Geometry: final body of the model. Coordinates: model frame, mm. Face numbers are marked on the shaded views. A direction names the side the tool comes from. Give positions to 0.01 mm unless a question says otherwise; leave off trailing zeros. Write each loop counter-clockwise with the first axis right and the second up, starting at its lowest first coordinate (ties: lowest second). Pieces come first, ordered by that corner, then holes. Notation, with made-up numbers: M 62.25,-10.75 L 93.25,-10.75 A28 ccw 93.25,14.25 Z; hole C -15,17.5 d7. An arc over 180 degrees is marked long. Use one line per item in the form item = value. Start each with the question number.
Item 1: Section query D-D on x = 15.75. Return loops of the section in (y, z).
Item 2: Access query for the marked faces 5, 6, 7, 8 and 9. Directions: +Z, -Z, +X, -X, +Y, -Y. A direction counts if a zero-diameter tool reaches every point of the face in a straight line with its end or side. Return the directions, or none.
Item 3: Section query C-C on x = 2.75. Return loops of the section in (y, z).
Item 4: Pull-direction query (X, two-part tool) for the marked faces 1, 2, 3 and 4; classes: released by +X, released by -X, zero draft, split by the parting line, or undercut.
Item 5: Contact query for flat-ended pins moving along their axis: P1, Ø1.5, axis at x = 16, z = 10.5, coming from the -Y side; P2, Ø7, axis at y = 10.5, z = 9, coming from the -X side; P3, Ø10.5, axis at y = 11, z = 10.5, coming from the +X side. Output: stop coordinate, or through.
Item 6: Material intervals for line 1 along X through (y, z) = (22.5, 4); line 2 along Y through (x, z) = (9.25, 3.25); line 3 along X through (y, z) = (7, 2) (3 decimals), sorted ascending. Write a range as from..to.
Item 7: Section query A-A on y = 23.5. Return loops of the section in (x, z), then the cut area to 3 significant figures.
from build123d import *

# Parameters (mm, degrees)
F0_W        = 7.366
F0_H        = 10.16
F1_DEPTH    = 19.05
F2_T4_DEPTH = 19.05
F2_T9_DEPTH = 19.05
F3_SIZE     = 2.54
F4_SIZE     = 6.35
F5_R        = 1.016


# Not quite as in the source:
# - a fillet or chamfer that OpenCascade refuses, or shapes differently, is made with other operations: its cross-section is extruded or revolved along the edge and cut away or added


with BuildPart() as f1:
    # F0 (on Top) → F1 (new body)
    with BuildSketch(Plane.XY):
        Polygon((0, 20.4722661398), (0, 0), (3.175, 0), (3.175, 10.16), (3.175, 11.43), (8.255, 11.43), (13.335, 11.43), (13.335, 0), (16.51, 0), (16.51, 20.4722661398), (19.3675, 20.4722661398), (19.3675, 33.02), (16.1925, 33.02), (16.1925, 20.32), (8.255, 20.32), (0.3175, 20.32), (0.3175, 33.02), (-2.8575, 33.02), (-2.8575, 20.4722661398), align=None)
        with Locations((6.858, 5.08)):
            Rectangle(F0_W, F0_H)
    extrude(amount=F1_DEPTH)

    # F2: chamfer of 5.08 on 2 edges, made by hand


with BuildPart() as f2_tool2:
    # F2_s3 → F2_t4 (new body)
    with BuildSketch(Plane.XY):
        Polygon((-5.08, 20.4722661398), (0, 15.3922661398), (0, 20.4722661398), align=None)
    extrude(amount=F2_T4_DEPTH)

    split(bisect_by=Plane.YZ.offset(-2.8575), keep=Keep.TOP)


with BuildPart() as f1_1:
    add(f1.part)

    # F2_t1: union F2_tool2
    add(f2_tool2.part)


with BuildPart() as f2_tool7:
    # F2_s8 → F2_t9 (new body)
    with BuildSketch(Plane.XY):
        Polygon((16.51, 15.3922661398), (21.59, 20.4722661398), (16.51, 20.4722661398), align=None)
    extrude(amount=F2_T9_DEPTH)

    split(bisect_by=Plane.YZ.offset(19.3675), keep=Keep.BOTTOM)


with BuildPart() as f1_2:
    add(f1_1.part)

    # F2_t6: union F2_tool7
    add(f2_tool7.part)

    # F3
    f3_edges = [f1_2.edges().sort_by_distance(p)[0] for p in [
        (16.51, 0, 9.525),
        (19.3675, 33.02, 9.525),
    ]]
    chamfer(f3_edges, length=F3_SIZE)

    # F4
    f4_edges = [f1_2.edges().sort_by_distance(p)[0] for p in [
        (0, 0, 9.525),
    ]]
    chamfer(f4_edges, length=F4_SIZE)

    # F5
    f5_edges = [f1_2.edges().sort_by_distance(p)[0] for p in [
        (13.335, 11.43, 9.525),
        (10.541, 10.16, 9.525),
    ]]
    fillet(f5_edges, radius=F5_R)


solid = f1_2.part
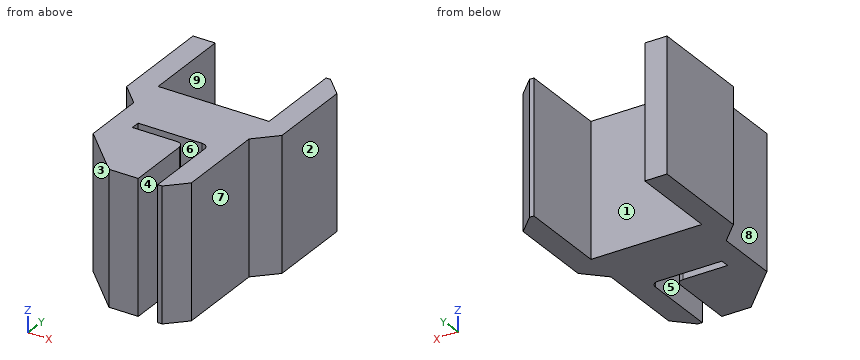
Answer sheet:
q1.outline = M 1.78,0 L 20.32,0 L 20.32,19.05 L 1.78,19.05 Z
q2.face_5 = +Z, -Z, -Y
q2.face_6 = +Z, -Z
q2.face_7 = +Z, -Z, +X, -Y
q2.face_8 = +Z, -Z, -X, -Y
q2.face_9 = +Z, -Z, +Y
q3.outline = M 3.6,0 L 20.32,0 L 20.32,19.05 L 3.6,19.05 Z
q4.face_1 = undercut
q4.face_2 = released by +X
q4.face_3 = released by -X
q4.face_4 = undercut
q5.P1 = 1.28
q5.P2 = 0
q5.P3 = 17.37
q6.line_1 = -2.86..0.32, 16.19..19.37
q6.line_2 = 0..10.16, 11.43..20.32
q6.line_3 = 0..10.541, 13.335..16.51
q7.outline = M -2.86,0 L 0.32,0 L 0.32,19.05 L -2.86,19.05 Z; M 16.19,0 L 19.37,0 L 19.37,19.05 L 16.19,19.05 Z
q7.area = 121 mm2
